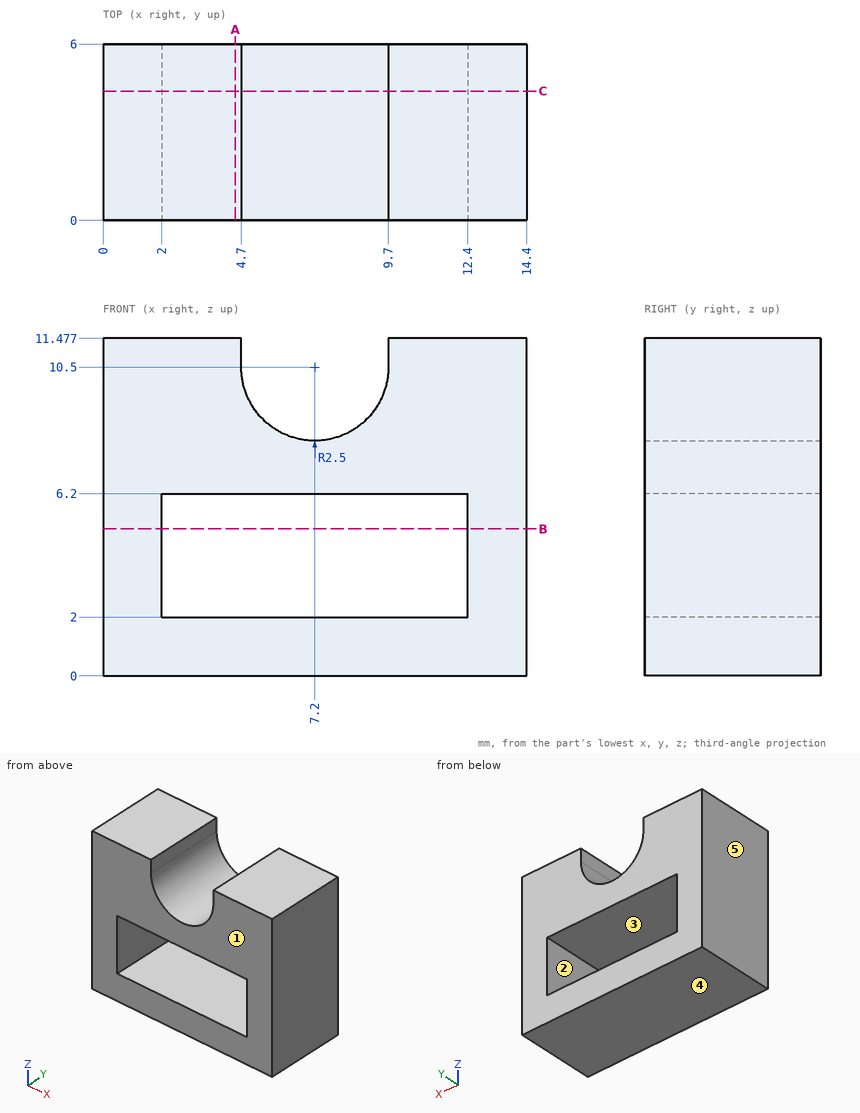
Input: dimensioned drawing with shaded views. Units: mm. Origin: part minimum x, y, z. A direction names the side the tool comes from. Coordinates: 2 decimals unless noted, no trailing zeros. Order: outer loops, then holes, each group sorted by start corner. A loop starts at its lowest first (then second) coordinate and runs counter-clockwise, first axis right, second up. Notation, with made-up numbers: M 74,9.25 L 131,9.25 A18 ccw 131,43.25 Z; hole C 46,9 d11. An arc over 180 degrees is marked long. Answer as CSV lines item,"result".
Q1. Section C-C on y = 4.4. Return the cut outline in (x, z), and give its area (3 significant figures).
Answers:
outline,"M 0,0 L 14.4,0 L 14.4,11.48 L 9.7,11.48 L 9.7,10.5 A2.5 cw 4.7,10.5 L 4.7,11.48 L 0,11.48 Z; hole M 2,2 L 12.4,2 L 12.4,6.2 L 2,6.2 Z"
area,"107 mm^2"
Q2. First-contact query: P1, Ø2, axis at x = 7, y = 4.5, coming from the +Z side; P2, Ø3, axis at x = 6.5, y = 2, coming from the +Z side. Flat tips, straight axial feed; report the tip coordinate or a pass-through.
Answers:
P1,"stops at z = 8.31"
P2,"stops at z = 9.31"
Q3. Section B-B on z = 5. Return the cut outline in (x, y), and give its area (3 significant figures).
Answers:
outline,"M 0,0 L 2,0 L 2,6 L 0,6 Z; M 12.4,0 L 14.4,0 L 14.4,6 L 12.4,6 Z"
area,"24.0 mm^2"
Q4. Line query: probe 1 along Z at (x, y) = (10.75, 5.75); probe 2 along X at (y, z) = (2, 2.25); probe 3 along Z at (x, y) = (5.75, 4.3). Output: solid intervals per line, ascending. Write a range as [from, to].
Answers:
probe 1,"z = [0, 2], [6.2, 11.48]"
probe 2,"x = [0, 2], [12.4, 14.4]"
probe 3,"z = [0, 2], [6.2, 8.46]"
Q5. Section A-A on x = 4.5. Return the cut outline in (y, z), and give its area (3 significant figures).
Answers:
outline,"M 0,0 L 6,0 L 6,2 L 0,2 Z; M 0,6.2 L 6,6.2 L 6,11.48 L 0,11.48 Z"
area,"43.7 mm^2"
Q6. Draft query along Z for the marked faces 3, 4 and 5. Return one class per face: pulls with the +Z half, pulls with the -Z half, needs draft (parallel to the pull), parting line crosses it, or undercut.
Answers:
face 3,"undercut"
face 4,"pulls with the -Z half"
face 5,"needs draft"
Q7. Set-up query: the marked faces 1 and 2. Return all of +Z, -Z, +X, -X, +Y, -Y with unobstructed straight access to the full face (end or side cutting, diameter ignored); none if empty.
Answers:
face 1,"+Z, -Z, +X, -X, -Y"
face 2,"+Y, -Y"
